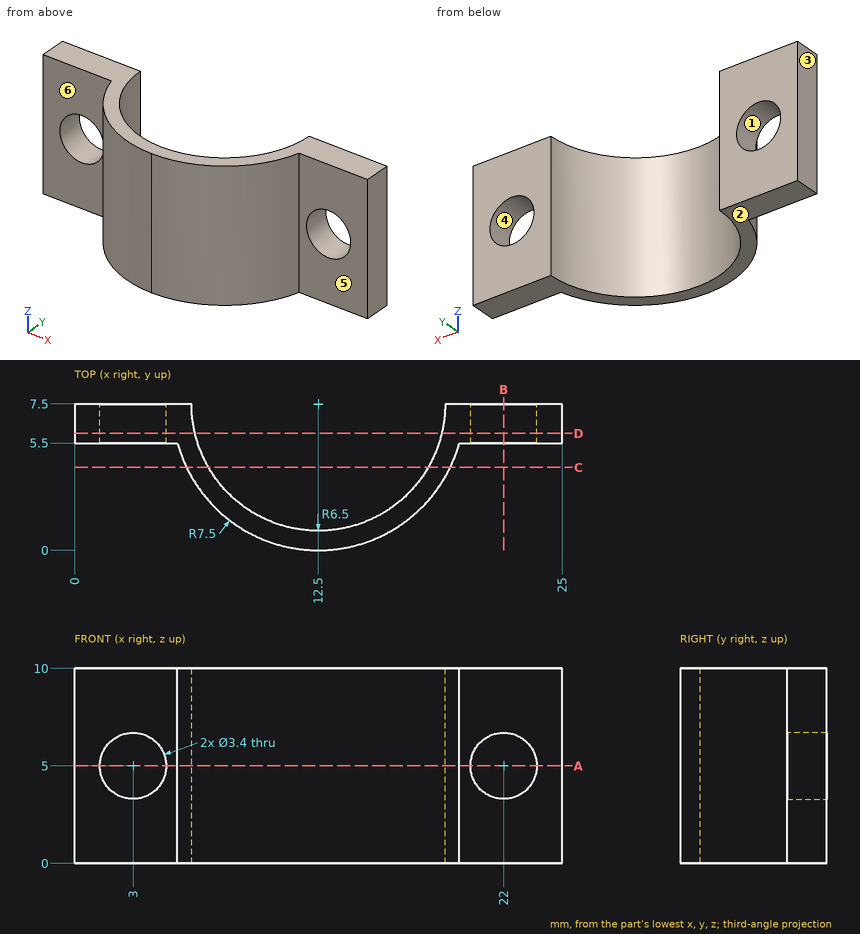
Design review of the part shown in the three views and the two pictorial views. Dimensions are in mm from the part's minimum x, y and z. A direction names the side the tool comes from. Give positions to 0.01 mm unless a question says otherwise; leave off trailing zeros. Loops run counter-clockwise (first coordinate to the right, second up) from the corner with the lowest first, then second, coordinate; pieces in that order, holes last. Notation, with made-up numbers: M 86.5,-16 L 93.5,-16 A20 ccw 93.5,15 Z; hole C -23.5,43 d6. An arc over 180 degrees is marked long. Answer as a JSON object with one key per item and string values.
Item 1: For P1, Ø4.5, axis at x = 3, z = 5, coming from the +Y side; P2, Ø4, axis at x = 11, z = 1.5, coming from the +Y side; P3, Ø1, axis at y = 4, z = 6, coming from the -X side; P4, Ø2.5, axis at x = 22, z = 5, coming from the -Y side, all flat-tipped, find the tip position at first contact; note any pin that passes through.
Output values:
{"P1": "stops at y = 7.5", "P2": "stops at y = 2.02", "P3": "stops at x = 5.63", "P4": "passes through"}
Item 2: Machinability: for the marked faces 4, 5 and 6, which of the approach directions +Z, -Z, +X, -X, +Y, -Y give a long, thin tool a straight path to every point of the face, cutting with its end or side? Answer none if there is none.
Output values:
{"face 4": "+Y, -Y", "face 5": "+Z, -Z, +X, -Y", "face 6": "+Z, -Z, -X, -Y"}
Item 3: We need section D-D (y = 6). State the section outline as (x, z) points, and give its area (3 significant figures).
Output values:
{"outline": "M 0,0 L 6.18,0 L 6.18,10 L 0,10 Z; M 18.82,0 L 25,0 L 25,10 L 18.82,10 Z; hole C 3,5 d3.4; hole C 22,5 d3.4", "area": "105 mm2"}
Item 4: We need section C-C (y = 4.25). State the section outline as (x, z) points.
Output values:
{"outline": "M 5.74,0 L 6.87,0 L 6.87,10 L 5.74,10 Z; M 18.13,0 L 19.26,0 L 19.26,10 L 18.13,10 Z"}
Item 5: Wall thickness on line 1 along X through (y, z) = (6.85, 5); line 2 along X through (y, z) = (5.75, 5.75); line 3 along X through (y, z) = (4.75, 1.5): over which ranges is each line inside the solid? List them lowest first.
Output values:
{"line 1": "x = 0 to 1.3, 4.7 to 6.03, 18.97 to 20.3, 23.7 to 25", "line 2": "x = 0 to 1.47, 4.53 to 6.24, 18.76 to 20.47, 23.53 to 25", "line 3": "x = 5.52 to 6.61, 18.39 to 19.48"}
Item 6: We need section A-A (z = 5). State the section outline as (x, y) points, and give its area (3 significant figures).
Output values:
{"outline": "M 0,5.5 L 1.3,5.5 L 1.3,7.5 L 0,7.5 Z; M 4.7,5.5 L 5.27,5.5 A7.5 ccw 19.73,5.5 L 20.3,5.5 L 20.3,7.5 L 19,7.5 A6.5 cw 6,7.5 L 4.7,7.5 Z; M 23.7,5.5 L 25,5.5 L 25,7.5 L 23.7,7.5 Z", "area": "28.8 mm2"}
Item 7: We need section B-B (x = 22). State the section outline as (y, z) points, and give its area (3 significant figures).
Output values:
{"outline": "M 5.5,0 L 7.5,0 L 7.5,3.3 L 5.5,3.3 Z; M 5.5,6.7 L 7.5,6.7 L 7.5,10 L 5.5,10 Z", "area": "13.2 mm2"}
Item 8: Mouldability with a two-part tool opening along X and no side actions: class the marked faces 1, 2 and 3 as pulls with the +X half, pulls with the -X half, needs draft (parallel to the pull), parting line crosses it, or undercut.
Output values:
{"face 1": "undercut", "face 2": "needs draft", "face 3": "pulls with the -X half"}
